```python
from build123d import *

# Parameters (mm, degrees)
EXTRUDE_1_DEPTH = 70
SHELL_1_T       = -1


with BuildPart() as part:
    # 草图1 → 凸台-拉伸1 (new body)
    with BuildSketch(Plane.XY):
        with BuildLine():
            Line((-90, -90), (90, -90))
            ThreePointArc((90, -90), (97.071067812, -87.071067812), (100, -80))
            Line((100, -80), (100, 80))
            ThreePointArc((100, 80), (97.071067812, 87.071067812), (90, 90))
            Line((90, 90), (-90, 90))
            ThreePointArc((-90, 90), (-97.071067812, 87.071067812), (-100, 80))
            Line((-100, 80), (-100, -80))
            ThreePointArc((-100, -80), (-97.071067812, -87.071067812), (-90, -90))
        make_face()
    extrude(amount=EXTRUDE_1_DEPTH)

    # 抽壳1
    shell_1_openings = [part.faces().sort_by_distance(p)[0] for p in [
        (0, 0, 70),
    ]]
    offset(amount=SHELL_1_T, openings=shell_1_openings, kind=Kind.INTERSECTION)


solid = part.part
```
Build history of the part. All positions in model axes, mm. A direction names the side the tool comes from. Round coordinates to 2 decimals unless told otherwise and drop trailing zeros. Loops run counter-clockwise (first coordinate to the right, second up) from the corner with the lowest first, then second, coordinate; pieces in that order, holes last.
Item 1: Saw through at B-B (y = 52.5). List the corners of the cut face in (x, z), then the cut area to 3 significant figures.
Item 2: Which spindle directions (+Z, -Z, +X, -X, +Y, -Y) get a long thin tool onto all of the face, cutting with end or side? Do faces 1 (the face through (-1, 1, 1)), 2 (the face through (96.99, -87.15, 34.51)). Say none if no direction does.
Item 3: Saw through at A-A (z = 14). List the corners of the cut face in (x, y).
Item 4: Pin check, flat tips, straight feed: P1, Ø10, axis at x = -73, y = 40.5, coming from the +Z side; P2, Ø2, axis at x = 79, y = 68.5, coming from the -Z side. Stop position of each tip, or through.
Item 5: Two-plate mould, pull along Y, no slides. Class faces 3 (the face through (-99, 1, 35)), 4 (the face through (-100, 1, 35)), 5 (the face through (97.15, 86.99, 34.51)): released by +Y, released by -Y, zero draft, split by the parting line, or undercut.
Item 6: Saw through at C-C (x = -32). List the corners of the cut face in (y, z).
Item 7: Drill centre lines: line 1 along Y through (x, z) = (-84.5, 30.5); line 2 along X through (y, z) = (-55, 56.5); line 3 along Z through (x, y) = (-2, -11.5). Where is each one in solid material? Low to high.
Worked answers:
1. outline: (-100, 0) - (100, 0) - (100, 70) - (99, 70) - (99, 1) - (-99, 1) - (-99, 70) - (-100, 70) - close
1. area: 338 mm2
2. face 1: +Z
2. face 2: +Z, -Z, +X, -Y
3. outline: (-100, -80) arc R10 ccw to (-90, -90) - (90, -90) arc R10 ccw to (100, -80) - (100, 80) arc R10 ccw to (90, 90) - (-90, 90) arc R10 ccw to (-100, 80) - close; hole (-99, -80) arc R9 ccw to (-90, -89) - (90, -89) arc R9 ccw to (99, -80) - (99, 80) arc R9 ccw to (90, 89) - (-90, 89) arc R9 ccw to (-99, 80) - close
4. P1: stops at z = 1
4. P2: stops at z = 0
5. face 3: undercut
5. face 4: zero draft
5. face 5: released by +Y
6. outline: (-90, 0) - (90, 0) - (90, 70) - (89, 70) - (89, 1) - (-89, 1) - (-89, 70) - (-90, 70) - close
7. line 1: y = -90 to -89, 89 to 90
7. line 2: x = -100 to -99, 99 to 100
7. line 3: z = 0 to 1
